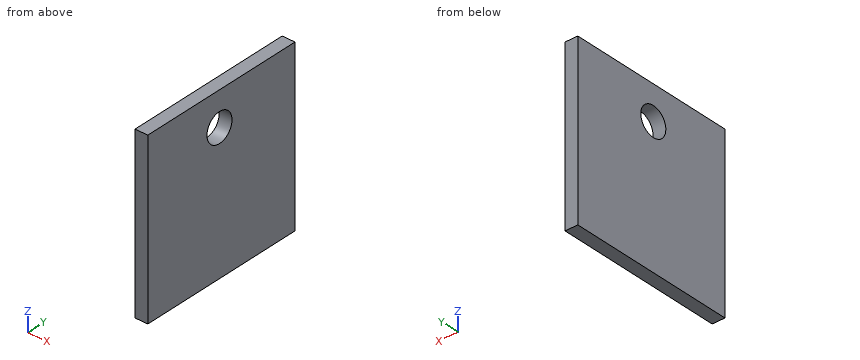
```python
from build123d import *

# Parameters (mm, degrees)
CYLINDER033_R     = 1.7
CYLINDER033_DEPTH = 20
BOX045_W          = 1.5
BOX045_H          = 20
BOX045_DEPTH      = 20


with BuildPart() as cylinder033:
    # Cylinder033 → Cylinder033 (new body)
    with BuildSketch(Plane(origin=(254, 19.74, 51.5), x_dir=(0, 0, -1), z_dir=(1, 0, 0))):
        Circle(CYLINDER033_R)
    extrude(amount=CYLINDER033_DEPTH)


with BuildPart() as testside_wall:
    # Box045 → Box045 (new body)
    with BuildSketch(Plane(origin=(254, 10, 35.5), x_dir=(1, 0, 0), z_dir=(0, 0, 1))):
        with Locations((0.75, 10)):
            Rectangle(BOX045_W, BOX045_H)
    extrude(amount=BOX045_DEPTH)

    # Cut054: cut Cylinder033
    add(cylinder033.part, mode=Mode.SUBTRACT)


solid = testside_wall.part
```
Can you work these out from the model? Positions are in its coordinate system, mm. Give positions to 0.01 mm unless a question says otherwise; leave off trailing zeros. Loops run counter-clockwise (first coordinate to the right, second up) from the corner with the lowest first, then second, coordinate; pieces in that order, holes last. Notation, with made-up numbers: M 84,81 L 111,81 A17 ccw 111,101 Z; hole C -0.5,23 d8. An arc over 180 degrees is marked long. Use CSV: the item, a comma, the result in double quotes. Start each with the question number.
1. Imagine slicing it at B-B, the plane z = 51.5. Write out the boundary of the cut face in (x, y).
2. If I drill on L1, parallel to Z at x = 255.05, y = 19.74; L2, parallel to Y at x = 254.4, z = 51.5; L3, parallel to Z at x = 255.2, y = 19, over which ranges is the centre line in solid material (lowest first)?
3. Imagine slicing it at C-C, the plane x = 254.7. Write out the boundary of the cut face in (y, z).
4. Imagine slicing it at A-A, the plane y = 19.74. Write out the boundary of the cut face in (x, z).
5. For P1, Ø2.5, axis at y = 19.74, z = 51.5, coming from the -X side, with a flat end and sliding along its axis, tell me the tip position at first contact or that it passes through.
Response values:
1,outline,"M 254,10 L 255.5,10 L 255.5,18.04 L 254,18.04 Z; M 254,21.44 L 255.5,21.44 L 255.5,30 L 254,30 Z"
2,L1,"35.5 to 49.8, 53.2 to 55.5"
2,L2,"10 to 18.04, 21.44 to 30"
2,L3,"35.5 to 49.97, 53.03 to 55.5"
3,outline,"M 10,35.5 L 30,35.5 L 30,55.5 L 10,55.5 Z; hole C 19.74,51.5 d3.4"
4,outline,"M 254,35.5 L 255.5,35.5 L 255.5,49.8 L 254,49.8 Z; M 254,53.2 L 255.5,53.2 L 255.5,55.5 L 254,55.5 Z"
5,P1,"through"
